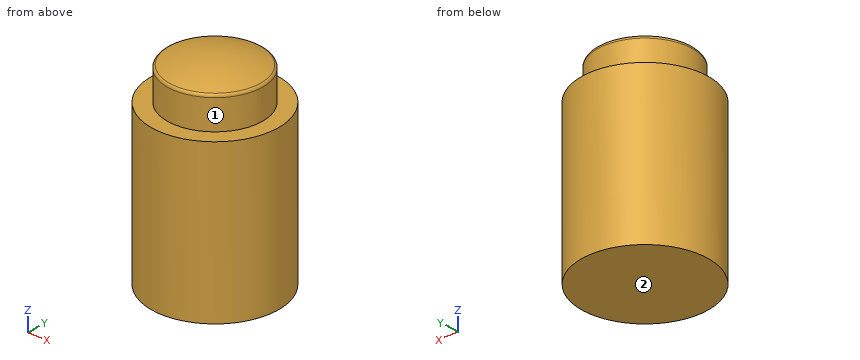
```python
from build123d import *

# Parameters (mm, degrees)
SKETCH1_R           = 30
BOSS_EXTRUDE1_DEPTH = 20
DOME1_FACE_RADIUS   = 30
DOME1_HEIGHT        = 7
SKETCH2_R           = 40
BOSS_EXTRUDE2_DEPTH = 100
FILLET1_R           = 2


with BuildPart() as part:
    # Sketch1 → Boss-Extrude1 (new body)
    with BuildSketch(Plane.XY):
        Circle(SKETCH1_R)
    extrude(amount=BOSS_EXTRUDE1_DEPTH)

    # Dome1: a dome of height H over a round flat face of radius A is a cap of a sphere of radius (A * A + H * H) / (2 * H)
    dome1_r = (DOME1_FACE_RADIUS * DOME1_FACE_RADIUS + DOME1_HEIGHT * DOME1_HEIGHT) / (2 * DOME1_HEIGHT)
    dome1_base = Plane((0, 0, 20), z_dir=(0, 0, 1))
    with Locations(dome1_base.offset(DOME1_HEIGHT - dome1_r)):
        dome1_ball = Sphere(dome1_r, mode=Mode.PRIVATE)
    add(split(dome1_ball, bisect_by=dome1_base, keep=Keep.TOP, mode=Mode.PRIVATE))

    # Sketch2 → Boss-Extrude2 (add)
    with BuildSketch(Plane(origin=(0, 0, 0), x_dir=(-1, 0, 0), z_dir=(0, 0, -1))):
        with Locations(Location((0, 0, 0), (0, 0, 180))):
            Circle(SKETCH2_R)
    extrude(amount=BOSS_EXTRUDE2_DEPTH)

    # Fillet1
    fillet1_edges = [part.edges().sort_by_distance(p)[0] for p in [
        (-30, 0, 20),
    ]]
    fillet(fillet1_edges, radius=FILLET1_R)


solid = part.part
```
The model under review builds one solid part; all positions refer to its coordinate system, in mm. Face numbers are marked on the shaded views. A direction names the side the tool comes from. Round coordinates to 2 decimals unless told otherwise and drop trailing zeros. Order: outer loops, then holes, each group sorted by start corner. A loop starts at its lowest first (then second) coordinate and runs counter-clockwise, first axis right, second up. Notation, with made-up numbers: (-35, 61.5) -> (6, 61.5) arc R31 ccw to (6, 96.5) -> close; hole circle Ø2 at (86, 41.5). An arc over 180 degrees is marked (long way). Use a Markdown table: item, result.
Q1. We need section A-A on z = -77. Write out the cut boundary in (x, y).
Values:
| item | result |
|---|---|
| outline | circle Ø80 at (0, 0) |
Q2. We need section B-B on x = 35. Write out the cut boundary in (y, z), then the cut area to 3 significant figures.
Values:
| item | result |
|---|---|
| outline | (-19.36, -100) -> (19.36, -100) -> (19.36, 0) -> (-19.36, 0) -> close |
| area | 3,870 mm^2 |
Q3. Tool access review of the marked faces 1 and 2: name each direction out of +Z, -Z, +X, -X, +Y, -Y from which nothing blocks a thin tool from reaching the whole face with its end or side.
Values:
| item | result |
|---|---|
| face 1 | +Z |
| face 2 | -Z, +X, -X, +Y, -Y |
Q4. For line 1 (Z direction, x = -19.5, y = -26.5); line 2 (X direction, y = -1.5, z = -92); line 3 (Y direction, x = 24, z = -6.5), list the stretches that pass through material, from the lowest coordinate up.
Values:
| item | result |
|---|---|
| line 1 | z = -100 to 0 |
| line 2 | x = -39.97 to 39.97 |
| line 3 | y = -32 to 32 |
Q5. Clearance check with flat-ended pins moving along their axes: P1, Ø8, axis at x = 4, z = -9.5, coming from the +Y side; P2, Ø12, axis at y = -1.5, z = -28.5, coming from the +X side; P3, Ø1.5, axis at y = 13.5, z = 8.5, coming from the -X side; P4, Ø6, axis at y = -14, z = -83.5, coming from the +X side. State where each tip first meets the part, or that it passes through.
Values:
| item | result |
|---|---|
| P1 | stops at y = 40 |
| P2 | stops at x = 40 |
| P3 | stops at x = -27.16 |
| P4 | stops at x = 38.46 |
